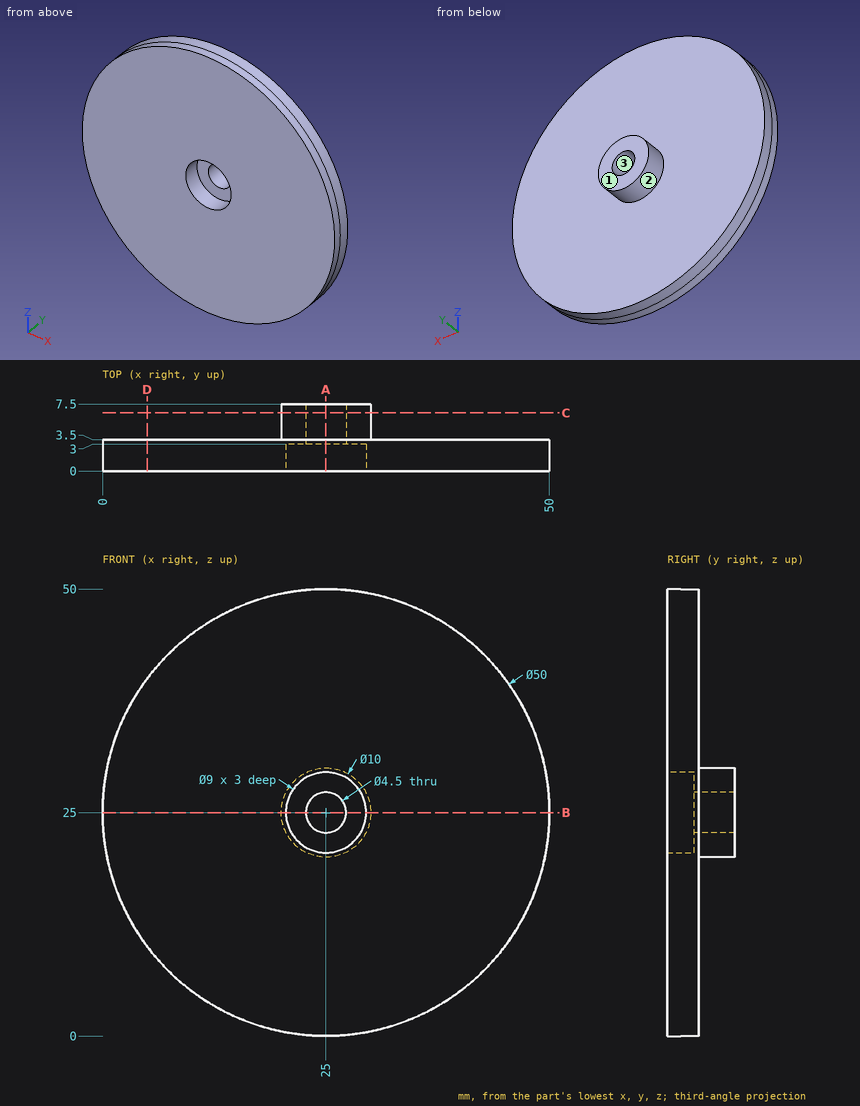
Print and shaded views of the part. All mm, measured from the part's lowest x, y and z. Give positions to 0.01 mm unless a question says otherwise; leave off trailing zeros. Write each loop counter-clockwise with the first axis right and the second up, starting at its lowest first coordinate (ties: lowest second). Pieces come first, ordered by that corner, then holes. Notation, with made-up numbers: (-5.75, 48) -> (9.25, 48) arc R24 ccw to (9.25, 79) -> close; hole circle Ø3 at (42.5, -4.5). An arc over 180 degrees is marked (long way). Use CSV: the item, a comma, the result in double quotes. Start each with the question number.
1) Pin check, flat tips, straight feed: P1, Ø2, axis at x = 24, z = 22.5, coming from the -Y side; P2, Ø4, axis at x = 38, y = 4, coming from the -Z side; P3, Ø1, axis at y = 3.5, z = 44.5, coming from the +X side. Stop position of each tip, or through.
2) Drill centre lines: L1, parallel to X at y = 0.6, z = 25; L2, parallel to X at y = 6.6, z = 25; L3, parallel to Y at x = 25.5, z = 11. Where is each one in solid material? Low to high.
3) Cut at D-D on x = 5. List the corners of the cut face in (y, z), plus the area to 3 significant figures.
4) Cut at B-B on z = 25. List the corners of the cut face in (x, y).
5) Cut at C-C on y = 6.5. List the corners of the cut face in (x, z).
6) Cut at A-A on x = 25. List the corners of the cut face in (y, z).
7) Two-plate mould, pull along Z, no slides. Class the marked faces 1, 2 and 3: released by +Z, released by -Z, zero draft, split by the parting line, or undercut.
Final values:
1,P1,"stops at y = 3"
1,P2,"stops at z = 2.58"
1,P3,"stops at x = 41.25"
2,L1,"x = 0 to 20.5, 29.5 to 50"
2,L2,"x = 20 to 22.75, 27.25 to 30"
2,L3,"y = 0 to 3.5"
3,outline,"(0, 10) -> (3.5, 10) -> (3.5, 40) -> (0, 40) -> close"
3,area,"105 mm2"
4,outline,"(0, 0) -> (20.5, 0) -> (20.5, 3) -> (22.75, 3) -> (22.75, 7.5) -> (20, 7.5) -> (20, 3.5) -> (0, 3.5) -> close; (27.25, 3) -> (29.5, 3) -> (29.5, 0) -> (50, 0) -> (50, 3.5) -> (30, 3.5) -> (30, 7.5) -> (27.25, 7.5) -> close"
5,outline,"circle Ø10 at (25, 25); hole circle Ø4.5 at (25, 25)"
6,outline,"(0, 0) -> (3.5, 0) -> (3.5, 20) -> (7.5, 20) -> (7.5, 22.75) -> (3, 22.75) -> (3, 20.5) -> (0, 20.5) -> close; (0, 29.5) -> (3, 29.5) -> (3, 27.25) -> (7.5, 27.25) -> (7.5, 30) -> (3.5, 30) -> (3.5, 50) -> (0, 50) -> close"
7,face 1,"zero draft"
7,face 2,"split by the parting line"
7,face 3,"undercut"
